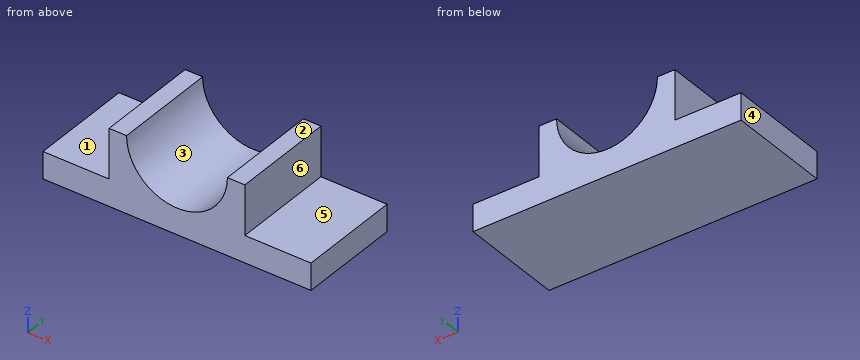
```python
from build123d import *

# Parameters (mm, degrees)
F0_W     = 193.04
F0_H     = 70.5103150129
F1_DEPTH = 147.32
F3_DEPTH = 25.4
F4_DEPTH = 147.32


with BuildPart() as f1:
    # F0 (on Front) → F1 (new body)
    with BuildSketch(Plane.XZ):
        Polygon((-190.5, -19.05), (190.5, -19.05), (190.5, 19.05), (96.52, 19.05), (-96.52, 19.05), (-190.5, 19.05), align=None)
        with Locations((0, 54.3051575065)):
            Rectangle(F0_W, F0_H)
    extrude(amount=F1_DEPTH)

    # F2 (on face) → F3 (cut)
    with BuildSketch(Plane.XZ.offset(147.32)):
        with BuildLine():
            ThreePointArc((-71.6898662242, 89.5603150129), (0, 17.8704487887), (71.6898662242, 89.5603150129))
            Line((71.6898662242, 89.5603150129), (-71.6898662242, 89.5603150129))
        make_face()
    extrude(amount=-F3_DEPTH, mode=Mode.SUBTRACT)

    # F4 (cut): a face of the model
    f4_faces = [f1.faces().sort_by_distance(p)[0] for p in [
        (0, -121.92, 59.1341908018),
    ]]
    extrude(f4_faces, amount=-F4_DEPTH, mode=Mode.SUBTRACT)


solid = f1.part
```
Read the model definition and answer for the solid it produces. Units are mm, in the model's axes. Face numbers are marked on the shaded views. A direction names the side the tool comes from. Coordinates: 2 decimals unless noted, no trailing zeros. Order: outer loops, then holes, each group sorted by start corner. A loop starts at its lowest first (then second) coordinate and runs counter-clockwise, first axis right, second up. Notation, with made-up numbers: (-23, 16) - (6, 16) arc R7 ccw to (6, 26) - close; hole circle Ø2 at (-35.75, 17.5). An arc over 180 degrees is marked (long way). Answer as a JSON object with one key per item and string values. Group by question number.
Item 1: The mould has two halves that part along X. Classify the marked faces 3, 4, 5 and 6: +X half, -X half, draft (parallel to the pull), parting line (faces both ways), or undercut.
Item 2: Section C-C (x = 0) is taken. Give the vertices of the cut face in (y, z).
Item 3: Section D-D (z = 71) is taken. Give the vertices of the cut face in (x, y), plus the area to 3 significant figures.
Item 4: Consider probe 1 along X at (y, z) = (-10, 85.5); probe 2 along Z at (x, y) = (136, -94); probe 3 along X at (y, z) = (-79, 74.5). Determine where each line is inside the solid, lowest interval first. Write a range as from..to.
Item 5: Section A-A (z = 38) is taken. Give the vertices of the cut face in (x, y).
Item 6: A tool of negligible diameter and unlimited length cuts with its end or side. For the marked faces 1 and 2, from which of +Z, -Z, +X, -X, +Y, -Y can it reach the whole face along a straight path? Write none if from no direction.
Item 7: Flat-ended cylindrical pins translate along their axes: P1, Ø4, axis at x = 129, z = 21, coming from the +Y side; P2, Ø1.5, axis at x = -65.5, y = -16.5, coming from the +Z side; P3, Ø12, axis at x = 35.5, y = -118.5, coming from the +Z side; P4, Ø5, axis at y = -120, z = 34, coming from the -X side. Find the tip coordinate at first contact, or state that the pin passes through.
Item 8: Section B-B (y = -100.5) is taken. Give the vertices of the cut face in (x, z), plus the area to 3 significant figures.
Results are:
{
 "1": {"face 3": "undercut", "face 4": "-X half", "face 5": "draft", "face 6": "+X half"},
 "2": {"outline": "(-147.32, -19.05) - (0, -19.05) - (0, 17.87) - (-147.32, 17.87) - close"},
 "3": {"outline": "(-96.52, -147.32) - (-69.25, -147.32) - (-69.25, 0) - (-96.52, 0) - close; (69.25, -147.32) - (96.52, -147.32) - (96.52, 0) - (69.25, 0) - close", "area": "8,040 mm^2"},
 "4": {"probe 1": "x = -96.52..-71.57, 71.57..96.52", "probe 2": "z = -19.05..19.05", "probe 3": "x = -96.52..-70.09, 70.09..96.52"},
 "5": {"outline": "(-96.52, -147.32) - (-49.81, -147.32) - (-49.81, 0) - (-96.52, 0) - close; (49.81, -147.32) - (96.52, -147.32) - (96.52, 0) - (49.81, 0) - close"},
 "6": {"face 1": "+Z, -X, +Y, -Y", "face 2": "+Z, +X, -X, +Y, -Y"},
 "7": {"P1": "stops at y = 0", "P2": "stops at z = 62.17", "P3": "stops at z = 31.1", "P4": "stops at x = -96.52"},
 "8": {"outline": "(-190.5, -19.05) - (190.5, -19.05) - (190.5, 19.05) - (96.52, 19.05) - (96.52, 89.56) - (71.69, 89.56) arc R71.69 cw to (-71.69, 89.56) - (-96.52, 89.56) - (-96.52, 19.05) - (-190.5, 19.05) - close", "area": "20,100 mm^2"}
}
